from build123d import *

# Parameters (mm, degrees)
BOSS_EXTRUDE1_DEPTH                                 = 12.7
CHAMFER1_SIZE2                                      = 47.397045256
CHAMFER1_SIZE                                       = 12.7
CSK_FOR_1_4_FLAT_HEAD_MACHINE_SCREW_100_D           = 7.14248
CSK_FOR_1_4_FLAT_HEAD_MACHINE_SCREW_100_CSINK_D     = 13.716
CSK_FOR_1_4_FLAT_HEAD_MACHINE_SCREW_100_CSINK_ANGLE = 100
LPATTERN1_COUNT                                     = 4
LPATTERN1_PITCH                                     = 457.2


with BuildPart() as part:
    # Sketch1 → Boss-Extrude1 (new body)
    with BuildSketch(Plane(origin=(0, 0, 0), x_dir=(1, 0, 0), z_dir=(0, 1, 0))):
        Polygon((-812.8, 0), (812.8, 0), (812.8, -292.1), (-1095.864592562, -292.1), align=None)
    extrude(amount=BOSS_EXTRUDE1_DEPTH)

    # Chamfer1
    chamfer1_edges = [part.edges().sort_by_distance(p)[0] for p in [
        (-141.532296281, 0, 292.1),
    ]]
    chamfer1_side = [part.faces().sort_by_distance(p)[0] for p in [
        (-141.532296281, 0.254, 292.1),
    ]]
    chamfer(chamfer1_edges, length=CHAMFER1_SIZE - 0.0001, length2=CHAMFER1_SIZE2 - 0.0001, reference=chamfer1_side[0])  # a hair under: the kernel refuses the full size

    # CSK for 1/4 Flat Head Machine Screw (100)1 (through all)
    with Locations(Plane(origin=(0, 12.7, 0), x_dir=(1, 0, 0), z_dir=(0, 1, 0))):
        with Locations((-685.8, -44.45), (-685.8, -196.85)):
            csk_for_1_4_flat_head_machine_screw_100 = CounterSinkHole(CSK_FOR_1_4_FLAT_HEAD_MACHINE_SCREW_100_D / 2, CSK_FOR_1_4_FLAT_HEAD_MACHINE_SCREW_100_CSINK_D / 2, counter_sink_angle=CSK_FOR_1_4_FLAT_HEAD_MACHINE_SCREW_100_CSINK_ANGLE)

    # LPattern1: CSK for 1/4 Flat Head Machine Screw (100)1 ×4
    with Locations(*[(i * LPATTERN1_PITCH, 0, 0) for i in range(1, LPATTERN1_COUNT)]):
        add(csk_for_1_4_flat_head_machine_screw_100, mode=Mode.SUBTRACT)


solid = part.part
Source: CAD feature listing. Evaluate the final solid. Frame: model axes, mm. Give positions to 0.01 mm unless a question says otherwise; leave off trailing zeros. Write each loop counter-clockwise with the first axis right and the second up, starting at its lowest first coordinate (ties: lowest second). Pieces come first, ordered by that corner, then holes. Notation, with made-up numbers: (81, 21) -> (121, 21) arc R20 cw to (121, 46) -> close; hole circle Ø7 at (-40, 83.25). An arc over 180 degrees is marked (long way). Return JSON: item names as keys, results as strings. Group by question number.
1. Material intervals for line 1 (X direction, y = 7.25, z = 196.85); line 2 (X direction, y = 7.25, z = 44.45); line 3 (Y direction, x = -882.5, z = 245), sorted ascending. Write a range as from..to.
2. Pin query (flat end, axial travel): pin 1 Ø2 at (y, z) = (9, 221.5) entering from -X; pin 2 Ø11.5 at (x, z) = (228.6, 44.45) entering from +Y; pin 3 Ø4.5 at (x, z) = (-685.8, 196.85) entering from +Y; pin 4 Ø8 at (x, z) = (685.8, 196.85) entering from +Y. Return the tip coordinate at first contact, or that it passes through.
3. Section B-B, the plane z = 266. Output: boundary loops of the cut face in (x, y).
4. Section C-C, the plane z = 71. Output: boundary loops of the cut face in (x, y), then the cut area to 3 significant figures.
Determined:
{
 "1": {"line 1": "x = -1003.56..-689.37, -682.23..-232.17, -225.03..225.03, 232.17..682.23, 689.37..812.8", "line 2": "x = -855.88..-689.37, -682.23..-232.17, -225.03..225.03, 232.17..682.23, 689.37..812.8", "line 3": "y = 0.08..12.7"},
 "2": {"pin 1": "stops at x = -1028.42", "pin 2": "stops at y = 11.77", "pin 3": "passes through", "pin 4": "stops at y = 10.3"},
 "3": {"outline": "(-1070.57, 5.71) -> (812.8, 5.71) -> (812.8, 12.7) -> (-1070.57, 12.7) -> close"},
 "4": {"outline": "(-881.6, 0) -> (812.8, 0) -> (812.8, 12.7) -> (-881.6, 12.7) -> close", "area": "21,500 mm2"}
}
